Autodesk Inventor part; units mm, degrees
ref_plane "YZ Plane" through (0, 0, 0) normal (1, 0, 0) x (0, 1, 0)
ref_plane "XZ Plane" through (0, 0, 0) normal (0, 1, 0) x (-1, 0, 0)
ref_plane "XY Plane" through (0, 0, 0) normal (0, 0, 1) x (1, 0, 0)
sketch "Sketch1" plane through (0, 0, 0) normal (0, 1, 0) x (-1, 0, 0)
  circle A0 centre (0, 0) radius 10
  dimension "d0" = 20
extrude "Extrusion1" add sketch "Sketch1" along normal blind 4
sketch "Sketch2" plane through (0, 4, 0) normal (0, 1, 0) x (1, 0, 0)
  line L0 (0, 0) -> (0, 6)
  circle A0 centre (0, 6) radius 2.125
  dimension "d3" = 6
  dimension "d4" = 4.25
extrude "Extrusion2" cut sketch "Sketch2" against normal through all
pattern_circular "Circular Pattern1" count 4 over 360 about axis through (0, 0, 0) along (0, 1, 0) of "Extrusion2"
sketch "Sketch3" plane through (0, 0, 0) normal (0, -1, 0) x (1, 0, 0)
  circle A0 centre (0, 0) radius 10
  arc A1 (-10, 0) -> (10, 0) centre (0, 0) ccw
  line L0 (10, 0) -> (10, -25)
  line L1 (10, -25) -> (-10, -25)
  line L2 (-10, -25) -> (-10, 0)
  dimension "d10" = 25
extrude "Extrusion3" add sketch "Sketch3" against normal blind 4 contours L0 L1 L2 A0
sketch "Sketch4" plane through (0, 4, 0) normal (0, 1, 0) x (1, 0, 0)
  line L0 (-10, 25) -> (-10, 0)
  line L1 (10, 25) -> (-10, 25)
  line L2 (-10, 25) -> (-10, 20)
  line L3 (-10, 20) -> (10, 20)
  line L4 (10, 20) -> (10, 25)
  point P0 (0, 0)
  dimension "d13" = 5
extrude "Extrusion4" add sketch "Sketch4" along normal blind 27
sketch "Sketch5" plane through (10, 0, -25) normal (0, 0, -1) x (-1, 0, 0)
  point P0 (10, 0)
sketch "Sketch6" plane through (10, 0, -25) normal (0, 0, -1) x (-1, 0, 0)
  line L0 (7.875, 4) -> (12.125, 4)
  line L1 (20, 31) -> (0, 31)
  line L2 (10, 17.5) -> (20, 17.5)
  line L3 (10, 17.5) -> (10, 23.5)
  line L4 (10, 23.5) -> (10, 25.5)
  circle A0 centre (10, 25.5) radius 2.125
  point P0 (10, 0)
  dimension "d16" = 6
  dimension "d26" = 2
  dimension "d27" = 4.25
extrude "Extrusion5" cut sketch "Sketch6" against normal through all
pattern_linear "Rectangular Pattern1" count 3 spacing 6 along (-1, 0, 0) count 2 spacing 18 along (0, -1, 0) of "Extrusion5" first direction both ways yes
sketch "Sketch7" plane through (-10, 4, -20) normal (0, 0, 1) x (1, 0, 0)
  circle A0 centre (10, 21.5) radius 2.125
  circle A1 centre (10, 3.5) radius 2.125
  line L0 (10, 21.5) -> (10, 3.5)
  line L1 (6, 7) -> (14, 7)
  line L2 (14, 7) -> (14, 18)
  line L3 (14, 18) -> (6, 18)
  line L4 (6, 18) -> (6, 7)
  line L5 (6, 7) -> (14, 18) construction
  line L6 (14, 7) -> (6, 18) construction
  point P0 (10, -4)
  point P1 (10, 12.5)
  dimension "d29" = 8
  dimension "d30" = 11
extrude "Extrusion6" cut sketch "Sketch7" against normal through all contours L3 L2 L1 L0 | L0 L1 L4 L3
properties part number "ClawJoint"
Can you work these out from the model? Positions are in its coordinate system, mm. A direction names the side the tool comes from. Round coordinates to 2 decimals unless told otherwise and drop trailing zeros. Write each loop counter-clockwise with the first axis right and the second up, starting at its lowest first coordinate (ties: lowest second). Pieces come first, ordered by that corner, then holes. Notation, with made-up numbers: (68.25, 57) -> (88.25, 57) arc R22 cw to (88.25, 95) -> close; hole circle Ø10 at (88, 21). An arc over 180 degrees is marked (long way). One line per question, with ' | ' between items. Start each with the question number.
1) On a 3-axis mill with a long thin cutter (end or side, diameter ignored), from which of +Z, -Z, +X, -X, +Y, -Y can I reach the whole of each face in a straight line? I mean faces 1 (the flat face through (0, 0, -11)), 2 (the flat face through (4, 16, -22)), 3 (the flat face through (4.3, 17.3, -20)). Say none if no direction works.
2) If we mould it in two halves opening along Z, with no side actions, what happens to faces 4 (the cylindrical face through (0, 2, 10)), 5 (the cylindrical face through (0.461, 5.426, -22.535)), 6 (the cylindrical face through (-3.926, 2.028, 0.461)), 7 (the cylindrical face through (-0.461, 2.028, -3.926))? For each: released by +Z, released by -Z, zero draft, split by the parting line, or undercut.
3) I need wall thicknesses on line 1 (X direction, y = 7.5, z = -22.95) (3 decimals); line 2 (Y direction, x = 0, z = -22.8) (3 decimals); line 3 (Y direction, x = 6, z = -22.7) (3 decimals). Which ranges of each line are inside material? Lowest first, please. Write a range as [from, to].
4) Suppose I cut it at A-A on x = 6. Write out the boundary of the cut face in (y, z) (3 decimals).
5) Suppose I cut it at C-C on x = 0. Write out the boundary of the cut face in (y, z) (3 decimals).
6) Suppose I cut it at B-B on y = 25.5. Write out the boundary of the cut face in (x, z) (3 decimals).
7) Suppose I cut it at D-D on z = -7. Write out the boundary of the cut face in (x, y) (3 decimals), then the cut area to 3 significant figures.
8) I'm going to push flat-ended pins straight in: P1, Ø5, axis at x = -2, y = 20.5, coming from the +Z side; P2, Ø10, axis at x = 2, z = 6, coming from the +Y side; P3, Ø4, axis at x = 0, y = 25.5, coming from the -Z side. Where does each tip first touch, or does it pass through?
Return value:
1) face 1: +Z, -Z, +X, -X, -Y | face 2: +Z, -Z | face 3: +Z, +X, -X, +Y
2) face 4: released by +Z | face 5: zero draft | face 6: undercut | face 7: undercut
3) line 1: x = [-10, -8.125], [-3.875, -2.125], [2.125, 3.875], [8.125, 10] | line 2: y = [0, 5.375], [9.625, 11], [22, 23.375], [27.625, 31] | line 3: y = [0, 5.375], [9.625, 23.375], [27.625, 31]
4) outline: (0, -25) -> (5.375, -25) -> (5.375, -20) -> (4, -20) -> (4, -2.125) -> (0, -2.125) -> close; (0, 2.125) -> (4, 2.125) -> (4, 8) -> (0, 8) -> close; (9.625, -25) -> (23.375, -25) -> (23.375, -20) -> (9.625, -20) -> close; (27.625, -25) -> (31, -25) -> (31, -20) -> (27.625, -20) -> close
5) outline: (0, -25) -> (5.375, -25) -> (5.375, -20) -> (4, -20) -> (4, -8.125) -> (0, -8.125) -> close; (0, -3.875) -> (4, -3.875) -> (4, 3.875) -> (0, 3.875) -> close; (0, 8.125) -> (4, 8.125) -> (4, 10) -> (0, 10) -> close; (9.625, -25) -> (11, -25) -> (11, -20) -> (9.625, -20) -> close; (22, -25) -> (23.375, -25) -> (23.375, -20) -> (22, -20) -> close; (27.625, -25) -> (31, -25) -> (31, -20) -> (27.625, -20) -> close
6) outline: (-10, -25) -> (-8.125, -25) -> (-8.125, -20) -> (-10, -20) -> close; (-3.875, -25) -> (-2.125, -25) -> (-2.125, -20) -> (-3.875, -20) -> close; (2.125, -25) -> (3.875, -25) -> (3.875, -20) -> (2.125, -20) -> close; (8.125, -25) -> (10, -25) -> (10, -20) -> (8.125, -20) -> close
7) outline: (-10, 0) -> (-1.875, 0) -> (-1.875, 4) -> (-10, 4) -> close; (1.875, 0) -> (10, 0) -> (10, 4) -> (1.875, 4) -> close | area: 65.0 mm2
8) P1: stops at z = -20 | P2: stops at y = 4 | P3: passes through
